Geometry: final body of the model. Coordinates: model frame, mm. Coordinates: 2 decimals unless noted, no trailing zeros. Loops run counter-clockwise (first coordinate to the right, second up) from the corner with the lowest first, then second, coordinate; pieces in that order, holes last. Notation, with made-up numbers: (-23.5, 35) - (34.5, 35) arc R13 cw to (34.5, 41) - close; hole circle Ø7 at (71.25, -16.5). An arc over 180 degrees is marked (long way). Put each result on its own line as item: value. Start each with the question number.
1) Material intervals for line 1 along Y through (x, z) = (-6.35, 2.05); line 2 along X through (y, z) = (171.45, 0.95); line 3 along Y through (x, z) = (23.5, 1.8), sorted ascending. Write a range as from..to.
2) Section C-C on x = 6.35. Output: boundary loops of the cut face in (y, z).
3) Contact query for a flat-ended pin moving along its axis: pin 1 Ø6 at (x, y) = (29, 157.5) entering from -Z. Output: stop coordinate, or through.
4) Section A-A on y = 57.15. Output: boundary loops of the cut face in (x, z).
5) Section D-D on y = 120.65. Output: boundary loops of the cut face in (x, z).
6) Section B-B on z = 1.85. Output: boundary loops of the cut face in (x, y), and give its area (3 significant figures).
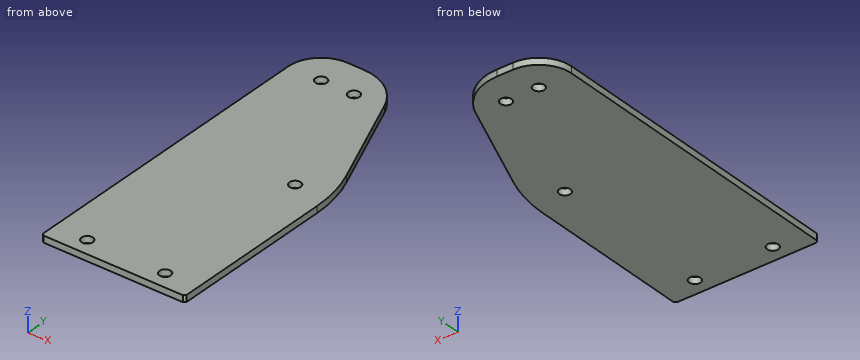
Autodesk Inventor part; units mm, degrees
ref_plane "YZ Plane" through (0, 0, 0) normal (1, 0, 0) x (0, 1, 0)
ref_plane "XZ Plane" through (0, 0, 0) normal (0, 1, 0) x (-1, 0, 0)
ref_plane "XY Plane" through (0, 0, 0) normal (0, 0, 1) x (1, 0, 0)
sketch "Sketch1" plane through (0, 0, 0) normal (0, 0, 1) x (1, 0, 0)
  circle A0 centre (-6.35, 171.45) radius 2.1844
  circle A1 centre (6.35, 171.45) radius 2.1844
  circle A2 centre (23.8125, 120.65) radius 2.1844
  circle A3 centre (23.8125, 57.15) radius 2.1844
  circle A4 centre (-6.35, 57.15) radius 2.1844
  line L0 (-19.05, 50.8) -> (36.5125, 50.8)
  line L1 (36.5125, 50.8) -> (36.5125, 125.2738)
  line L2 (36.5125, 125.2738) -> (12.725, 184.15)
  line L3 (12.725, 184.15) -> (-19.05, 184.15)
  line L4 (-19.05, 184.15) -> (-19.05, 50.8)
  point P0 (0, 0)
  dimension "d0" = 12.7
  dimension "d2" = 12.7
  dimension "d3" = 6.35
  dimension "d4" = 12.7
  dimension "d5" = 63.5
  dimension "d6" = 112
extrude "Extrusion1" add sketch "Sketch1" along normal blind 2.54
fillet "Fillet1" radius 12.7 1 edges at (-19.05, 184.15, 1.27)
fillet "Fillet2" radius 19.05 1 edges at (12.725, 184.15, 1.27)
fillet "Fillet3" radius 50.8 1 edges at (36.5125, 125.2738, 1.27)
chamfer "Chamfer1" distance 0.7937 angle 45 2 edges at (36.5125, 50.8, 1.27) (-19.05, 50.8, 1.27)
properties part number "funnelFront" material "white pla"
Answer block:
1. line 1: y = 50.8..54.97, 59.33..169.27, 173.63..184.15
1. line 2: x = -19.05..-8.53, -4.17..4.17, 8.53..17.86
1. line 3: y = 50.8..54.99, 59.31..118.49, 122.81..157.48
2. outline: (50.8, 0) - (169.27, 0) - (169.27, 2.54) - (50.8, 2.54) - close; (173.63, 0) - (183.02, 0) - (183.02, 2.54) - (173.63, 2.54) - close
3. pin 1: passes through
4. outline: (-19.05, 0) - (-8.53, 0) - (-8.53, 2.54) - (-19.05, 2.54) - close; (-4.17, 0) - (21.63, 0) - (21.63, 2.54) - (-4.17, 2.54) - close; (26, 0) - (36.51, 0) - (36.51, 2.54) - (26, 2.54) - close
5. outline: (-19.05, 0) - (21.63, 0) - (21.63, 2.54) - (-19.05, 2.54) - close; (26, 0) - (36.24, 0) - (36.24, 2.54) - (26, 2.54) - close
6. outline: (-19.05, 51.59) - (-18.26, 50.8) - (35.72, 50.8) - (36.51, 51.59) - (36.51, 115.4) arc R50.8 ccw to (32.81, 134.43) - (17.54, 172.24) arc R19.05 ccw to (-0.12, 184.15) - (-6.35, 184.15) arc R12.7 ccw to (-19.05, 171.45) - close; hole circle Ø4.37 at (-6.35, 57.15); hole circle Ø4.37 at (-6.35, 171.45); hole circle Ø4.37 at (6.35, 171.45); hole circle Ø4.37 at (23.81, 57.15); hole circle Ø4.37 at (23.81, 120.65)
6. area: 6,560 mm²
